The listing builds one solid part. Answer for the finished solid, in the listing's coordinates (mm). A direction names the side the tool comes from. Give positions to 0.01 mm unless a question says otherwise; leave off trailing zeros. Order: outer loops, then holes, each group sorted by start corner. A loop starts at its lowest first (then second) coordinate and runs counter-clockwise, first axis right, second up. Notation, with made-up numbers: (2, -28) -> (51, -28) arc R36 cw to (51, 9) -> close; hole circle Ø2 at (70.25, -35.75). An arc over 180 degrees is marked (long way). Write item = value, one per line. Start each with the question number.
```python
from build123d import *

# Parameters (mm, degrees)
BOSS_EXTRUDE1_DEPTH = 5.08


with BuildPart() as part:
    # Sketch1 → Boss-Extrude1 (new body)
    with BuildSketch(Plane(origin=(0, 0, 0), x_dir=(1, 0, 0), z_dir=(0, 1, 0))):
        Polygon((-127, 0), (0, 127), (127, 0), (0, -127), align=None)
        with BuildLine():
            ThreePointArc((7.065247253, -50.947438662), (36.37003729, -36.37003729), (50.947438662, -7.065247253))
            ThreePointArc((50.947438662, -7.065247253), (53.066892499, -3.148903914), (57.237245905, -1.5875))
            Line((57.237245905, -1.5875), (114.910495706, -1.5875))
            Line((114.910495706, -1.5875), (114.910495706, 1.5875))
            Line((114.910495706, 1.5875), (57.237245905, 1.5875))
            ThreePointArc((57.237245905, 1.5875), (53.066892499, 3.148903914), (50.947438662, 7.065247253))
            ThreePointArc((50.947438662, 7.065247253), (36.37003729, 36.37003729), (7.065247253, 50.947438662))
            ThreePointArc((7.065247253, 50.947438662), (3.148903914, 53.066892499), (1.5875, 57.237245905))
            Line((1.5875, 57.237245905), (1.5875, 114.910495706))
            Line((1.5875, 114.910495706), (-1.5875, 114.910495706))
            Line((-1.5875, 114.910495706), (-1.5875, 57.237245905))
            ThreePointArc((-1.5875, 57.237245905), (-3.148903914, 53.066892499), (-7.065247253, 50.947438662))
            ThreePointArc((-7.065247253, 50.947438662), (-36.37003729, 36.37003729), (-50.947438662, 7.065247253))
            ThreePointArc((-50.947438662, 7.065247253), (-53.066892499, 3.148903914), (-57.237245905, 1.5875))
            Line((-57.237245905, 1.5875), (-114.910495706, 1.5875))
            Line((-114.910495706, 1.5875), (-114.910495706, -1.5875))
            Line((-114.910495706, -1.5875), (-57.237245905, -1.5875))
            ThreePointArc((-57.237245905, -1.5875), (-53.066892499, -3.148903914), (-50.947438662, -7.065247253))
            ThreePointArc((-50.947438662, -7.065247253), (-36.37003729, -36.37003729), (-7.065247253, -50.947438662))
            ThreePointArc((-7.065247253, -50.947438662), (-3.148903914, -53.066892499), (-1.5875, -57.237245905))
            Line((-1.5875, -57.237245905), (-1.5875, -114.910495706))
            Line((-1.5875, -114.910495706), (1.5875, -114.910495706))
            Line((1.5875, -114.910495706), (1.5875, -57.237245905))
            ThreePointArc((1.5875, -57.237245905), (3.148903914, -53.066892499), (7.065247253, -50.947438662))
        make_face(mode=Mode.SUBTRACT)
    extrude(amount=BOSS_EXTRUDE1_DEPTH)


solid = part.part
```
Item 1: A cutting plane is placed at A-A, the plane z = -78. Write down the section's boundary in (x, y).
Item 2: Flat-ended cylindrical pins translate along their axes: pin 1 (1.5 mm diameter, centred on x = -100, y = 2, fed in from -Z); pin 2 (2.5 mm diameter, centred on x = 0, y = 2, fed in from -Z); pin 3 (2.5 mm diameter, centred on x = 0, y = 3.5, fed in from +Z). Find the tip coordinate at first contact, or state that the pin passes through.
Item 3: A cutting plane is placed at B-B, the plane x = 111. Write down the section's boundary in (y, z).
Item 4: Which of the six approach directions +Z, -Z, +X, -X, +Y, -Y give full straight-line access (tool end or side, diameter ignored) to faces 1 (the flat face through (58, 0, -2)), 2 (the cylindrical face through (-36.039, 2.504, -36.698))?
Item 5: Consider L1, parallel to Z at x = 38, y = 1.25; L2, parallel to Z at x = 87.5, y = 0.2; L3, parallel to X at y = 2.85, z = -42. Determine where each line is inside the solid, lowest interval first. Write a range as from..to.
Item 6: The mould has two halves that part along X. Classify faces 3 (the flat face through (63, 3, -64)), 4 (the flat face through (58, 5.08, -2)), 5 (the cylindrical face through (36.039, 2.504, 36.698)): +X half, -X half, draft (parallel to the pull), parting line (faces both ways), or undercut.
Check values:
q1.outline = (-49, 0) -> (-1.59, 0) -> (-1.59, 5.08) -> (-49, 5.08) -> close; (1.59, 0) -> (49, 0) -> (49, 5.08) -> (1.59, 5.08) -> close
q2.pin_1 = -27.75
q2.pin_2 = -127
q2.pin_3 = 127
q3.outline = (0, -16) -> (5.08, -16) -> (5.08, -1.59) -> (0, -1.59) -> close; (0, 1.59) -> (5.08, 1.59) -> (5.08, 16) -> (0, 16) -> close
q4.face_1 = +Z, -Z, +X, -X, -Y
q4.face_2 = +Y, -Y
q5.L1 = -89..-34.66, 34.66..89
q5.L2 = -39.5..-1.59, 1.59..39.5
q5.L3 = -85..-29.69, 29.69..85
q6.face_3 = +X half
q6.face_4 = draft
q6.face_5 = undercut
